For this review, use the dimensioned drawing (mm, ordinates from the lowest corner) and the shaded views. A direction names the side the tool comes from. Give positions to 0.01 mm unless a question says otherwise; leave off trailing zeros. Write each loop counter-clockwise with the first axis right and the second up, starting at its lowest first coordinate (ties: lowest second). Pieces come first, ordered by that corner, then holes.
1) We need section B-B on y = 42. Give the boundary of the cut face in (x, z).
2) We need section C-C on x = 10.5. Give the boundary of the cut face in (y, z), and give its area (3 significant figures).
3) Draft analysis for pull direction Y (two halves, no side actions). For the marked faces 1, 2 and 3, state which applies: pulls with the +Y half, pulls with the -Y half, needs draft (parallel to the pull), parting line crosses it, or undercut.
4) For P1, Ø1, axis at x = 24, y = 11.5, coming from the +Z side, flat-tipped, find the tip position at first contact; note if it passes through.
5) Machinability: for the marked faces 4 and 5, which of the approach directions +Z, -Z, +X, -X, +Y, -Y give a long, thin tool a straight path to every point of the face, cutting with its end or side? Answer none if there is none.
6) We need section A-A on z = 2.65. Give the boundary of the cut face in (x, y), and give its area (3 significant figures).
7) Wall thickness on line 1 along X through (y, z) = (26, 3.85); line 2 along Y through (x, z) = (23, 2.6); line 3 along Z through (x, y) = (16, 44): over which ranges is each line inside the solid? List them lowest first.
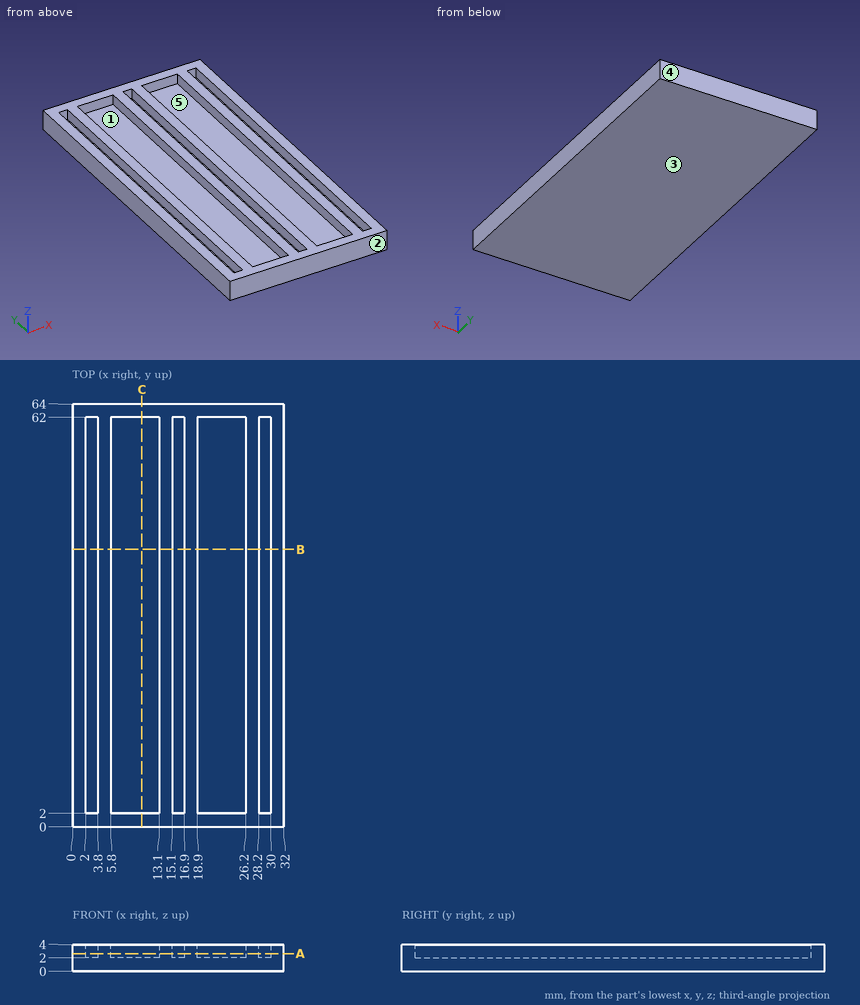
Results list:
1. outline: (0, 0) - (32, 0) - (32, 4) - (30, 4) - (30, 2) - (28.2, 2) - (28.2, 4) - (26.2, 4) - (26.2, 2) - (18.9, 2) - (18.9, 4) - (16.9, 4) - (16.9, 2) - (15.1, 2) - (15.1, 4) - (13.1, 4) - (13.1, 2) - (5.8, 2) - (5.8, 4) - (3.8, 4) - (3.8, 2) - (2, 2) - (2, 4) - (0, 4) - close
2. outline: (0, 0) - (64, 0) - (64, 4) - (62, 4) - (62, 2) - (2, 2) - (2, 4) - (0, 4) - close
2. area: 136 mm2
3. face 1: undercut
3. face 2: pulls with the -Y half
3. face 3: needs draft
4. P1: stops at z = 2
5. face 4: +Z, -Z, +X, -X, +Y
5. face 5: +Z
6. outline: (0, 0) - (32, 0) - (32, 64) - (0, 64) - close; hole (2, 2) - (3.8, 2) - (3.8, 62) - (2, 62) - close; hole (5.8, 2) - (13.1, 2) - (13.1, 62) - (5.8, 62) - close; hole (15.1, 2) - (16.9, 2) - (16.9, 62) - (15.1, 62) - close; hole (18.9, 2) - (26.2, 2) - (26.2, 62) - (18.9, 62) - close; hole (28.2, 2) - (30, 2) - (30, 62) - (28.2, 62) - close
6. area: 848 mm2
7. line 1: x = 0 to 2, 3.8 to 5.8, 13.1 to 15.1, 16.9 to 18.9, 26.2 to 28.2, 30 to 32
7. line 2: y = 0 to 2, 62 to 64
7. line 3: z = 0 to 2
